```python
from build123d import *

# Parameters (mm, degrees)
CUT_EXTRUDE1_DEPTH      = 31.245937227
CUT_EXTRUDE1_DEPTH_BACK = 31.245937227
SKETCH2_R               = 3.175
CHAMFER1_SIZE           = 0.635
CHAMFER1_SIZE_2         = 1.705739105


with BuildPart() as part:
    # Sketch1 → Revolve1 (revolve)
    with BuildSketch(Plane.XY, mode=Mode.PRIVATE) as revolve1_sk:
        with BuildLine():
            Line((17.4625, -17.4625), (17.4625, -13.894606786))
            ThreePointArc((17.4625, -13.894606786), (11.560204499, -8.032687253), (9.398, 0))
            Line((9.398, 0), (0, 0))
            Line((0, 0), (0, -17.4625))
            Line((0, -17.4625), (17.4625, -17.4625))
        make_face()
    revolve(revolve1_sk.sketch.rotate(Axis((0, 0, 0), (0, 1, 0)), 90), axis=Axis((0, 0, 0), (0, 1, 0)))

    # Sketch2 → Cut-Extrude1 (cut, two sides: drawn at the far end of the back side and taken through both)
    with BuildSketch(Plane(origin=(0, 0, 0), x_dir=(1, 0, 0), z_dir=(0, 1, 0)).offset(-CUT_EXTRUDE1_DEPTH_BACK)):
        with Locations(Location((0, 0, 0), (0, 0, 270))):
            Circle(SKETCH2_R)
    extrude(amount=CUT_EXTRUDE1_DEPTH + CUT_EXTRUDE1_DEPTH_BACK, mode=Mode.SUBTRACT)

    # Chamfer1
    # the kernel refuses this chamfer: 1.705739105, 0.635 mm, written as the material it takes off along each edge
    with BuildSketch(Plane(origin=(0, 0, 0), x_dir=(0, 0, 1), z_dir=(-1, 0, 0))) as chamfer1_piece_1:
        Polygon((3.175, -CHAMFER1_SIZE), (3.175 + CHAMFER1_SIZE, 0), (3.175, 0), align=None)
    revolve(axis=Axis((0, 0, 0), (0, 1, 0)), mode=Mode.SUBTRACT)
    with BuildSketch(Plane(origin=(0, -17.4625, 0), x_dir=(0, 0, 1), z_dir=(-1, 0, 0))) as chamfer1_piece_2:
        Polygon((3.175 + CHAMFER1_SIZE, 0), (3.175, CHAMFER1_SIZE), (3.175, 0), align=None)
    revolve(axis=Axis((0, -17.4625, 0), (0, 1, 0)), mode=Mode.SUBTRACT)
    with BuildSketch(Plane(origin=(0, -17.4625, 0), x_dir=(0, 0, -1), z_dir=(1, 0, 0))) as chamfer1_piece_3:
        Polygon((17.4625, CHAMFER1_SIZE), (17.4625 - CHAMFER1_SIZE, 0), (17.4625, 0), align=None)
    revolve(axis=Axis((0, -17.4625, 0), (0, 1, 0)), mode=Mode.SUBTRACT)
    with BuildSketch(Plane(origin=(0, 0, 0), x_dir=(0, 0, -1), z_dir=(1, 0, 0))) as chamfer1_piece_4:
        with BuildLine():
            Line((9.411131055, -0.648131055), (9.398 - CHAMFER1_SIZE, 0))
            Line((9.398 - CHAMFER1_SIZE, 0), (9.398, 0))
            ThreePointArc((9.398, 0), (9.401471415, -0.333297329), (9.411131055, -0.648131055))
        make_face()
    revolve(axis=Axis((0, 0, 0), (0, 1, 0)), mode=Mode.SUBTRACT)
    with BuildSketch(Plane(origin=(0, -13.894606786, 0), x_dir=(0, 0, -1), z_dir=(1, 0, 0))) as chamfer1_piece_5:
        with BuildLine():
            Line((17.4625, -CHAMFER1_SIZE_2), (16.906238382, 0.332895332))
            ThreePointArc((16.906238382, 0.332895332), (17.161543174, 0.176303935), (17.4625, 0))
            Line((17.4625, 0), (17.4625, -CHAMFER1_SIZE_2))
        make_face()
    revolve(axis=Axis((0, -13.894606786, 0), (0, 1, 0)), mode=Mode.SUBTRACT)


solid = part.part
```
Geometry: final body of the model. Coordinates: model frame, mm. Round coordinates to 2 decimals unless told otherwise and drop trailing zeros. Write each loop counter-clockwise with the first axis right and the second up, starting at its lowest first coordinate (ties: lowest second). Pieces come first, ordered by that corner, then holes. Notation, with made-up numbers: (23, -32.75) -> (43, -32.75) arc R23 cw to (43, -14.75) -> close; hole circle Ø8 at (32, -9.75). An arc over 180 degrees is marked (long way). Return JSON: item names as keys, results as strings.
Q1. Section C-C on y = -8. Return the cut outline in (x, z) (3 decimals).
From the geometry:
{"outline": "circle Ø23.083 at (0, 0); hole circle Ø6.35 at (0, 0)"}
Q2. First-contact query: pin 1 Ø2 at (x, z) = (11.5, 10.5) entering from +Y; pin 2 Ø2 at (y, z) = (-10.5, 11.5) entering from +X; pin 3 Ø1.5 at (y, z) = (-7, 2) entering from -X. Flat tips, straight axial feed; report the tip coordinate or a pass-through.
From the geometry:
{"pin 1": "y = -11.78", "pin 2": "x = 8.9", "pin 3": "x = -11.24"}
Q3. Mould query, pull axis Z, two halves, no side actions, for faces 1 (the cylindrical face through (17, -16, 4)), 2 (the flat face through (-4, -17.462, 0)), 3 (the cylindrical face through (-1.93, -8.84, -2.52)). Classes: +Z half, -Z half, draft (parallel to the pull), parting line (faces both ways), or undercut.
From the geometry:
{"face 1": "parting line", "face 2": "draft", "face 3": "undercut"}
Q4. Section D-D on y = -3.5. Return the cut outline in (x, z) (3 decimals).
From the geometry:
{"outline": "circle Ø19.571 at (0, 0); hole circle Ø6.35 at (0, 0)"}
Q5. Section B-B on z = 0. Return the cut outline in (x, y) (1 decimal), and give its area (3 significant figures).
From the geometry:
{"outline": "(-17.5, -16.8) -> (-16.8, -17.5) -> (-3.8, -17.5) -> (-3.2, -16.8) -> (-3.2, -0.6) -> (-3.8, 0) -> (-8.8, 0) -> (-9.4, -0.6) arc R16 cw to (-16.9, -13.6) -> (-17.5, -15.6) -> close; (3.2, -16.8) -> (3.8, -17.5) -> (16.8, -17.5) -> (17.5, -16.8) -> (17.5, -15.6) -> (16.9, -13.6) arc R16 cw to (9.4, -0.6) -> (8.8, 0) -> (3.8, 0) -> (3.2, -0.6) -> close", "area": "337 mm2"}
Q6. Section A-A on x = 0. Return the cut outline in (y, z) (1 decimal), and give its area (3 significant figures).
From the geometry:
{"outline": "(-17.5, -16.8) -> (-16.8, -17.5) -> (-15.6, -17.5) -> (-13.6, -16.9) arc R16 cw to (-0.6, -9.4) -> (0, -8.8) -> (0, -3.8) -> (-0.6, -3.2) -> (-16.8, -3.2) -> (-17.5, -3.8) -> close; (-17.5, 3.8) -> (-16.8, 3.2) -> (-0.6, 3.2) -> (0, 3.8) -> (0, 8.8) -> (-0.6, 9.4) arc R16 cw to (-13.6, 16.9) -> (-15.6, 17.5) -> (-16.8, 17.5) -> (-17.5, 16.8) -> close", "area": "337 mm2"}
Q7. Ray query, line 1 (X direction, y = -15, z = 2.5); line 2 (Z direction, x = -2.5, y = -9.5); line 3 (X direction, y = -9.25, z = 0) (3 decimals). Return the intervals inside material, ascending.
From the geometry:
{"line 1": "-17.12 to -1.96, 1.96 to 17.12", "line 2": "-12.27 to -1.96, 1.96 to 12.27", "line 3": "-12.342 to -3.175, 3.175 to 12.342"}
